from build123d import *

# Parameters (mm, degrees)
CROQUIS1_R              = 2.5
SALIENTE_EXTRUIR1_DEPTH = 20
CROQUIS2_W              = 45
CROQUIS2_H              = 20.08756727
SALIENTE_EXTRUIR2_DEPTH = 10
CROQUIS3_R              = 2.5
SALIENTE_EXTRUIR3_DEPTH = 110


with BuildPart() as part:
    # Croquis1 → Saliente-Extruir1 (new body)
    with BuildSketch(Plane(origin=(0, 0, 0), x_dir=(1, 0, 0), z_dir=(0, 1, 0))):
        Circle(CROQUIS1_R)
    extrude(amount=SALIENTE_EXTRUIR1_DEPTH)

    # Croquis2 → Saliente-Extruir2 (add)
    with BuildSketch(Plane.XZ):
        with Locations((12.5, -0.043783635)):
            Rectangle(CROQUIS2_W, CROQUIS2_H)
    extrude(amount=SALIENTE_EXTRUIR2_DEPTH)

    # Croquis3 → Saliente-Extruir3 (add)
    with BuildSketch(Plane(origin=(0, 20, 0), x_dir=(1, 0, 0), z_dir=(0, 1, 0))):
        Circle(CROQUIS3_R)
    extrude(amount=SALIENTE_EXTRUIR3_DEPTH)


solid = part.part
Verification items for the finished model (mm, model axes). A direction names the side the tool comes from. Round coordinates to 2 decimals unless told otherwise and drop trailing zeros. Write each loop counter-clockwise with the first axis right and the second up, starting at its lowest first coordinate (ties: lowest second). Pieces come first, ordered by that corner, then holes.
(1) Section check C-C (y = 19). Enter the section's corners in (x, z).
Returned:
outline: circle Ø5 at (0, 0)
(2) Depth check by flat-ended pin: pin 1 Ø6 at (x, y) = (-3.5, 26) entering from +Z; pin 2 Ø3 at (x, z) = (6.5, -4) entering from +Y; pin 3 Ø5 at (x, y) = (0, 112.5) entering from +Z. Enter the tip coordinate at first touch or a pass-through.
Returned:
pin 1: stops at z = 2.45
pin 2: stops at y = 0
pin 3: stops at z = 2.5
(3) Access from +Z, -Z, +X, -X, +Y, -Y to the whole of each face (thin tool, end or side, straight path). Record for faces 1 (the flat face through (12, -5, -10.088)), 2 (the cylindrical face through (-0.54, 64.09, 2.44)).
Returned:
face 1: -Z, +X, -X, +Y, -Y
face 2: +Y
(4) Section check A-A (z = 0). Enter the section's corners in (x, y), plus the area to 3 significant figures.
Returned:
outline: (-10, -10) - (35, -10) - (35, 0) - (2.5, 0) - (2.5, 130) - (-2.5, 130) - (-2.5, 0) - (-10, 0) - close
area: 1,100 mm2
(5) Material ranges on line 1 (Y direction, x = 31, z = -5.75); line 2 (X direction, y = 34, z = 0); line 3 (X direction, y = 97, z = -0.5), recorded low to high.
Returned:
line 1: y = -10 to 0
line 2: x = -2.5 to 2.5
line 3: x = -2.45 to 2.45
(6) Section check B-B (x = 0). Enter the section's corners in (y, z).
Returned:
outline: (-10, -10.09) - (0, -10.09) - (0, -2.5) - (130, -2.5) - (130, 2.5) - (0, 2.5) - (0, 10) - (-10, 10) - close
